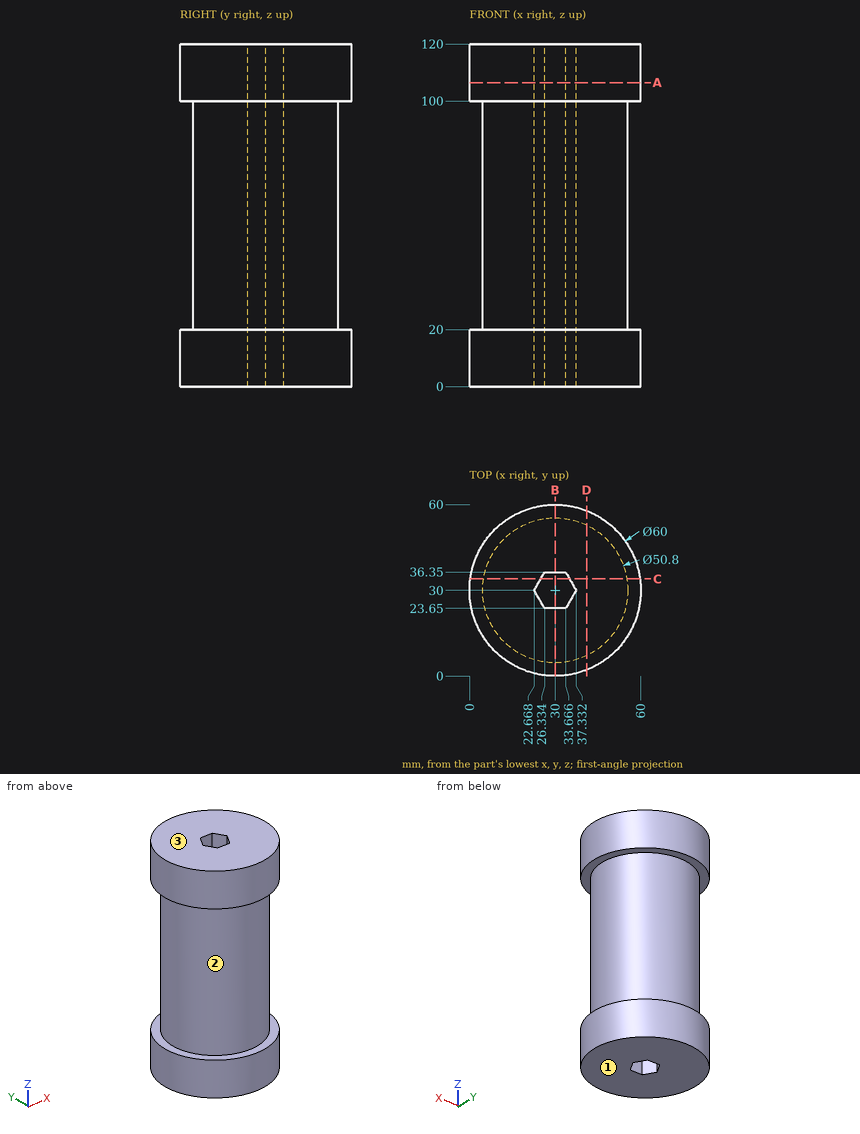
The drawing under review shows one solid part. Ordinate dimensions are in mm from its lowest x, y, z. Give positions to 0.01 mm unless a question says otherwise; leave off trailing zeros. Write each loop counter-clockwise with the first axis right and the second up, starting at its lowest first coordinate (ties: lowest second). Pieces come first, ordered by that corner, then holes.
1. Add section A-A, the plane z = 106.5. Write out the cut boundary in (x, y), plus the area to 3 significant figures.
2. Add section D-D, the plane x = 41. Write out the cut boundary in (y, z) (1 decimal), plus the area to 3 significant figures.
3. Add section C-C, the plane y = 34. Write out the cut boundary in (x, z), plus the area to 3 significant figures.
4. Add section B-B, the plane x = 30. Write out the cut boundary in (y, z).
5. For P1, Ø4, axis at y = 43, z = 43.5, coming from the -X side (1 decimal); P2, Ø1, axis at y = 29.5, z = 83, coming from the -X side; P3, Ø1.5, axis at x = 31.5, z = 76, coming from the -Y side, all flat-tipped, find the tip position at first contact; note any pin that passes through.
6. Draft analysis for pull direction Z (two halves, no side actions). For the marked faces 1, 2 and 3, state which applies: +Z half, -Z half, draft (parallel to the pull), parting line (faces both ways), or undercut.
7. Wall thickness on L1, parallel to Z at x = 5, y = 18; L2, parallel to Y at x = 24.5, z = 24 (1 decimal); L3, parallel to Y at x = 24, z = 51.5 (1 decimal): over which ranges is each line inside the solid? List them lowest first.
Worked answers:
1. outline: circle Ø60 at (30, 30); hole (22.67, 30) - (26.33, 23.65) - (33.67, 23.65) - (37.33, 30) - (33.67, 36.35) - (26.33, 36.35) - close
1. area: 2,690 mm2
2. outline: (2.1, 0) - (57.9, 0) - (57.9, 20) - (52.9, 20) - (52.9, 100) - (57.9, 100) - (57.9, 120) - (2.1, 120) - (2.1, 100) - (7.1, 100) - (7.1, 20) - (2.1, 20) - close
2. area: 5,900 mm2
3. outline: (0.27, 0) - (24.98, 0) - (24.98, 120) - (0.27, 120) - (0.27, 100) - (4.92, 100) - (4.92, 20) - (0.27, 20) - close; (35.02, 0) - (59.73, 0) - (59.73, 20) - (55.08, 20) - (55.08, 100) - (59.73, 100) - (59.73, 120) - (35.02, 120) - close
3. area: 5,190 mm2
4. outline: (0, 0) - (23.65, 0) - (23.65, 120) - (0, 120) - (0, 100) - (4.6, 100) - (4.6, 20) - (0, 20) - close; (36.35, 0) - (60, 0) - (60, 20) - (55.4, 20) - (55.4, 100) - (60, 100) - (60, 120) - (36.35, 120) - close
5. P1: stops at x = 7.1
5. P2: stops at x = 4.6
5. P3: stops at y = 4.61
6. face 1: -Z half
6. face 2: undercut
6. face 3: +Z half
7. L1: z = 0 to 20, 100 to 120
7. L2: y = 5.2 to 26.8, 33.2 to 54.8
7. L3: y = 5.3 to 27.7, 32.3 to 54.7
